Source: CAD feature listing. Evaluate the final solid. Frame: model axes, mm. A direction names the side the tool comes from. Round coordinates to 2 decimals unless told otherwise and drop trailing zeros. Order: outer loops, then holes, each group sorted by start corner. A loop starts at its lowest first (then second) coordinate and runs counter-clockwise, first axis right, second up. Notation, with made-up numbers: (21.25, 76) -> (80.25, 76) arc R21 ccw to (80.25, 81) -> close; hole circle Ø6 at (29.25, -2). An arc over 180 degrees is marked (long way). Write item = value, one per line. Start each with the question number.
(1) Draft query along Y for faces 1 (the face through (-3.4, 231.14, 10.3)), 2 (the face through (0.1, 7, -10.2)), 3 (the face through (12.932, 112.388, 5.362)). Return one class per face: released by +Y, released by -Y, zero draft, split by the parting line, or undercut.
(2) Cut plane B-B on y = 101.5. Return the cut outline in (x, z), then the cut area to 3 significant figures.
(3) Reachability of faces 4 (the face through (-2.38, 0.52, 10.74)), 5 (the face through (11.923, 119.03, -3.755)), 6 (the face through (12, 0, 8)), 7 (the face through (-2.17, 4.54, 9.76)), 8 (the face through (6, -6, 14)) from +Z, -Z, +X, -X, +Y, -Y: full face, straight path, thin tool, end or side. Return the list, or none.
(4) Contact query for flat-ended pins moving along their axis: pin 1 Ø3 at (x, y) = (5.5, 86.5) entering from -Z; pin 2 Ø6 at (x, z) = (5, 7) entering from -Y; pin 3 Ø12 at (y, z) = (175, 5) entering from -X. Output: stop coordinate, or through.
(5) Ray query, line 1 (X direction, y = 96, z = 0); line 2 (Z direction, x = 0, y = 3.7). Return the intervals inside material, ascending.
from build123d import *


with BuildPart() as part:
    # Sketch1 → Revolve1 (revolve)
    with BuildSketch(Plane.XY):
        with BuildLine():
            Line((12.5, 7), (12.5, 227.966923077))
            ThreePointArc((12.5, 227.966923077), (11.964906619, 229.258752773), (10.673076923, 229.793846154))
            Line((10.673076923, 229.793846154), (10, 230.466923077))
            Line((10, 230.466923077), (10.673076923, 231.14))
            Line((10.673076923, 231.14), (11.673076923, 231.14))
            ThreePointArc((11.673076923, 231.14), (13.355924313, 229.934344496), (14, 227.966923077))
            Line((14, 227.966923077), (14, 0))
            Line((14, 0), (15.5, 0))
            Line((15.5, 0), (15.5, -6))
            Line((15.5, -6), (14.5, -6))
            ThreePointArc((14.5, -6), (13.538055577, -2.948361096), (11, -1))
            Line((11, -1), (11, 2))
            Line((11, 2), (10, 2))
            Line((10, 2), (10, 7))
            Line((10, 7), (12.5, 7))
        make_face()
    revolve(axis=Axis((0, -1085.204253018, 0), (0, 1, 0)))


solid = part.part
Evaluation:
q1.face_1 = released by +Y
q1.face_2 = undercut
q1.face_3 = zero draft
q2.outline = circle Ø28 at (0, 0); hole circle Ø25 at (0, 0)
q2.area = 125 mm^2
q3.face_4 = -Y
q3.face_5 = none
q3.face_6 = +Y
q3.face_7 = +Y, -Y
q3.face_8 = +Z, -Z, +X, -X, -Y
q4.pin_1 = -13.42
q4.pin_2 = -1.26
q4.pin_3 = -14
q5.line_1 = -14 to -12.5, 12.5 to 14
q5.line_2 = -14 to -10, 10 to 14
